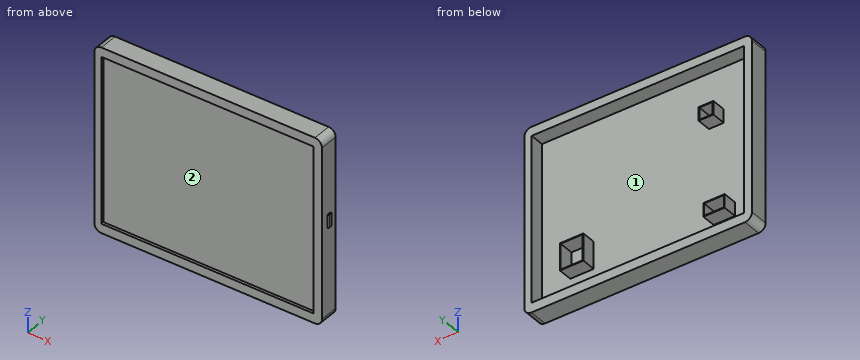
from build123d import *

# Parameters (mm, degrees)
F0_W      = 1600
F0_H      = 1295
F1_DEPTH  = 132
F2_R      = 50
F4_W      = 1491.3636445999
F4_H      = 1164.5535230637
F5_DEPTH  = 20
F7_W      = 1491.3636445999
F7_H      = 1164.5535230637
F8_DEPTH  = 100
F10_W     = 150
F10_H     = 95
F10_W_2   = 103.7647128105
F10_H_2   = 95.1176285744
F10_W_3   = 165
F10_H_3   = 190
F11_DEPTH = 100
F12_T     = -5
F13_W     = 30.2646905184
F13_H     = 95.1176509261
F14_DEPTH = 8
F15_R     = 5


# Not quite as in the source:
# - the program builds the solid bodies; features that only make, move or delete a surface that nothing else refers to are left out


with BuildPart() as f1:
    # F0 (on Front) → F1 (new body)
    with BuildSketch(Plane.XZ):
        with Locations((5.5797146633, 0)):
            Rectangle(F0_W, F0_H)
    extrude(amount=F1_DEPTH)

    # F2
    f2_edges = [f1.edges().sort_by_distance(p)[0] for p in [
        (-794.420285, -66, 647.5),
        (805.579715, -66, 647.5),
        (805.579715, -66, -647.5),
        (-794.420285, -66, -647.5),
    ]]
    fillet(f2_edges, radius=F2_R)

    # F4 (on offset) → F5 (cut)
    with BuildSketch(Plane.XZ.offset(132)):
        Rectangle(F4_W, F4_H)
    extrude(amount=-F5_DEPTH, mode=Mode.SUBTRACT)

    # F7 (on offset) → F8 (cut)
    with BuildSketch(Plane(origin=(0, 0, 0), x_dir=(-1, 0, 0), z_dir=(0, 1, 0))):
        with Locations((-8.7735056877, 2.2042393684)):
            Rectangle(F7_W, F7_H)
    extrude(amount=-F8_DEPTH, mode=Mode.SUBTRACT)

    # F10 (on offset) → F11 (join)
    with BuildSketch(Plane(origin=(0, -100, 0), x_dir=(-1, 0, 0), z_dir=(0, 1, 0))):
        with Locations((527.2952914238, -438.8382136822)):
            Rectangle(F10_W, F10_H)
        with Locations((471.1775481701, 244.2793995142)):
            Rectangle(F10_W_2, F10_H_2)
        with Locations((-473.1311607361, -343.8382136822)):
            Rectangle(F10_W_3, F10_H_3)
    extrude(amount=F11_DEPTH)

    # F12
    f12_openings = [f1.faces().sort_by_distance(p)[0] for p in [
        (-527.295291, 0, -438.838214),
        (-471.177548, 0, 244.2794),
        (473.131161, 0, -343.838214),
    ]]
    offset(amount=F12_T, openings=f12_openings, kind=Kind.INTERSECTION)

    # F13 (on face) → F14 (join)
    with BuildSketch(Plane.YZ.offset(805.5797146633)):
        with Locations((-62.757357955, 54.0441162884)):
            Rectangle(F13_W, F13_H)
    extrude(amount=F14_DEPTH)

    # F15
    f15_edges = [f1.edges().sort_by_distance(p)[0] for p in [
        (809.579715, -47.625013, 101.602942),
        (809.579715, -77.889703, 101.602942),
        (809.579715, -77.889703, 6.485291),
        (809.579715, -47.625013, 6.485291),
        (813.579715, -62.757358, 101.602942),
        (813.579715, -77.889703, 54.044116),
        (813.579715, -47.625013, 54.044116),
        (813.579715, -62.757358, 6.485291),
    ]]
    fillet(f15_edges, radius=F15_R)


solid = f1.part
For this review, take the finished solid that the model builds, in its own axes (mm). Face numbers are marked on the shaded views. Round coordinates to 2 decimals unless told otherwise and drop trailing zeros. Loops run counter-clockwise (first coordinate to the right, second up) from the corner with the lowest first, then second, coordinate; pieces in that order, holes last. Notation, with made-up numbers: (54, 63) - (99, 63) arc R20 cw to (99, 96) - close; hole circle Ø10 at (87.25, 72). An arc over 180 degrees is marked (long way). Use one line per item in the form item = value.
Item 1: Consider section A-A on x = 106. Write out the cut boundary in (y, z).
Answers:
outline = (-132, -647.5) - (0, -647.5) - (0, -580.07) - (-100, -580.07) - (-100, 584.48) - (0, 584.48) - (0, 647.5) - (-132, 647.5) - (-132, 582.28) - (-112, 582.28) - (-112, -582.28) - (-132, -582.28) - close; hole (-127, -642.5) - (-5, -642.5) - (-5, -585.07) - (-105, -585.07) - (-105, 589.48) - (-5, 589.48) - (-5, 642.5) - (-127, 642.5) - (-127, 587.28) - (-107, 587.28) - (-107, -587.28) - (-127, -587.28) - close
Item 2: Clearance check with flat-ended pins moving along their axes: P1, Ø5, axis at x = 182.5, z = -334.5, coming from the -Y side; P2, Ø1.5, axis at x = 806.5, y = -58.5, coming from the +Z side; P3, Ø5, axis at y = -22.5, z = 515.5, coming from the +X side. State where each tip first meets the part, or that it passes through.
Answers:
P1 = -112
P2 = 101.6
P3 = 805.58
Item 3: For line 1 (X direction, y = -31, z = 428); line 2 (Z direction, x = -425, y = -122); line 3 (Z direction, x = 100, y = -103), list the stretches that pass through material, from the lowest coordinate up.
Answers:
line_1 = -794.42 to -789.42, -741.91 to -736.91, 754.46 to 759.46, 800.58 to 805.58
line_2 = -647.5 to -642.5, -587.28 to -582.28, 582.28 to 587.28, 642.5 to 647.5
line_3 = -647.5 to -642.5, -585.07 to 589.48, 642.5 to 647.5
Item 4: Mouldability with a two-part tool opening along X and no side actions: class the marked faces 1 and 2 as +X half, -X half, draft (parallel to the pull), parting line (faces both ways), or undercut.
Answers:
face_1 = undercut
face_2 = undercut
